Here's how the part is built. I have some questions about the finished solid (model axes, mm). A direction names the side the tool comes from. Coordinates: 2 decimals unless noted, no trailing zeros. Write each loop counter-clockwise with the first axis right and the second up, starting at its lowest first coordinate (ties: lowest second). Pieces come first, ordered by that corner, then holes.
Autodesk Fusion 360 part; units mm, degrees
sketch "Sketch1" plane through (0, 0, 0) normal (0, 0, 1) x (1, 0, 0)
  line L0 (0, 0) -> (47.5, 0)
  line L1 (47.5, 0) -> (47.5, 38)
  circle A0 centre (5, 33) radius 2.175
  line L2 (5, 33) -> (5, 26) construction
  circle A1 centre (5, 26) radius 2.25
  circle A2 centre (12.5, 26) radius 2.25
  circle A3 centre (12.5, 33) radius 2.175
  circle A4 centre (20, 26) radius 2.25
  circle A5 centre (20, 33) radius 2.175
  line L3 (5, 26) -> (5, 19) construction
  line L4 (5, 19) -> (5, 12) construction
  circle A6 centre (5, 19) radius 2.325
  circle A7 centre (5, 12) radius 2.4
  circle A8 centre (12.5, 19) radius 2.325
  circle A9 centre (12.5, 12) radius 2.4
  circle A10 centre (20, 19) radius 2.325
  circle A11 centre (20, 12) radius 2.4
  circle A12 centre (27.5, 26) radius 2.25
  circle A13 centre (27.5, 33) radius 2.175
  circle A14 centre (27.5, 19) radius 2.325
  circle A15 centre (27.5, 12) radius 2.4
  circle A16 centre (35, 26) radius 2.25
  circle A17 centre (35, 33) radius 2.175
  circle A18 centre (35, 19) radius 2.325
  circle A19 centre (35, 12) radius 2.4
  line L5 (5, 12) -> (5, 5) construction
  circle A20 centre (5, 5) radius 2.475
  circle A21 centre (12.5, 5) radius 2.475
  circle A22 centre (20, 5) radius 2.475
  circle A23 centre (27.5, 5) radius 2.475
  circle A24 centre (35, 5) radius 2.475
  circle A25 centre (42.5, 26) radius 2.25
  circle A26 centre (42.5, 33) radius 2.175
  circle A27 centre (42.5, 19) radius 2.325
  circle A28 centre (42.5, 12) radius 2.4
  circle A29 centre (42.5, 5) radius 2.475
  line L6 (47.5, 38) -> (0, 38)
  line L7 (0, 38) -> (0, 0)
  dimension "d2" = 4.35
  dimension "d4" = 4.5
  dimension "d7" = 7.5
  dimension "d8" = 0
  dimension "d13" = 4.65
  dimension "d14" = 4.8
  dimension "d21" = 4.95
  dimension "d27" = 5
  dimension "d28" = 5
  dimension "d29" = 5
  dimension "d30" = 5
sketch "Sketch2" plane through (0, 0, 0) normal (0, 0, 1) x (1, 0, 0)
  line L0 (47.5, 0) -> (47.5, 38)
  line L1 (0, 0) -> (47.5, 0)
  line L2 (47.5, 38) -> (0, 38)
  line L3 (0, 38) -> (0, 0)
extrude "Extrude1" add sketch "Sketch2" against normal blind 8
extrude "Extrude2" cut sketch "Sketch1" against normal blind 5.8 contours A0 | A1 | A6
extrude "Extrude3" cut sketch "Sketch1" against normal blind 5.8 draft -2 contours A2 | A3 | A8 | A9
extrude "Extrude4" cut sketch "Sketch1" against normal blind 5.7 draft -4 contours A4 | A5 | A10 | A11 | A22
extrude "Extrude5" cut sketch "Sketch1" against normal blind 5.8 draft -6 contours A12 | A14 | A15 | A23
extrude "Extrude6" cut sketch "Sketch1" against normal blind 5.8 draft -8 contours A18 | A19 | A24
extrude "Extrude7" cut sketch "Sketch1" against normal blind 5.8 draft -10 contours A28 | A29
fillet "Fillet1" radius 3 3 edges at (0, 0, -4) (47.5, 0, -4) (47.5, 38, -4)
equation "extrude_depth = 5.8 mm"
1) Will these pins go through, and if not, where does the flat tip stop? pin 1 (1.3 mm diameter, centred on x = 5.5, y = 26, fed in from +Z); pin 2 (6 mm diameter, centred on x = 12.5, y = 26.5, fed in from +Z); pin 3 (2 mm diameter, centred on x = 20, y = 5.5, fed in from +Z).
Values follow:
pin 1: stops at z = -5.8
pin 2: stops at z = 0
pin 3: stops at z = -5.7
2) I need wall thicknesses on probe 1 along Y at (x, z) = (5, -4) (3 decimals); probe 2 along Y at (x, z) = (44, -4.25); probe 3 along Z at (x, y) = (21, 18). Which ranges of each line are inside material? Lowest first, please.
Values follow:
probe 1: y = 0 to 16.675, 21.325 to 23.75, 28.25 to 30.825, 35.175 to 38
probe 2: y = 0 to 4.15, 5.85 to 11.31, 12.69 to 38
probe 3: z = -8 to -5.7
3) We'd pull the mould along X, two halves only. Please class faces 3 (the face through (5, 26, -5.8)), 4 (the face through (46.6, 37.14, -4.06)), 5 (the face through (27.061, 17.024, -2.859)): pulls with the +X half, pulls with the -X half, needs draft (parallel to the pull), parting line crosses it, or undercut.
Values follow:
face 3: undercut
face 4: pulls with the +X half
face 5: undercut
4) Imagine slicing it at C-C on z = -2. Count the separate pieces of the cut face and the enclosed holes in it, then the cut area to 3 significant figures.
Values follow:
separate pieces: 1
enclosed holes: 21
area: 1,490 mm2
5) Imagine slicing it at A-A on y = 5. Please give me the cut outline in (x, z) (3 decimals), then the cut area to 3 significant figures.
Values follow:
outline: (0, -8) - (47.5, -8) - (47.5, 0) - (44.975, 0) - (43.952, -5.8) - (41.048, -5.8) - (40.025, 0) - (37.475, 0) - (36.66, -5.8) - (33.34, -5.8) - (32.525, 0) - (29.975, 0) - (29.365, -5.8) - (25.635, -5.8) - (25.025, 0) - (22.475, 0) - (22.076, -5.7) - (17.924, -5.7) - (17.525, 0) - (0, 0) - close
area: 282 mm2
6) Imagine slicing it at D-D on y = 33. Please give me the cut outline in (x, z) (3 decimals).
Values follow:
outline: (0, -8) - (47.5, -8) - (47.5, 0) - (22.175, 0) - (21.776, -5.7) - (18.224, -5.7) - (17.825, 0) - (14.675, 0) - (14.472, -5.8) - (10.528, -5.8) - (10.325, 0) - (7.175, 0) - (7.175, -5.8) - (2.825, -5.8) - (2.825, 0) - (0, 0) - close
7) On a 3-axis mill with a long thin cutter (end or side, diameter ignored), from which of +Z, -Z, +X, -X, +Y, -Y can I reach the whole of each face in a straight line? I mean faces 1 (the face through (47.5, 19, -4)), 2 (the face through (10.85, 31.74, -2.86)). Say none if no direction works.
Values follow:
face 1: +Z, -Z, +X, +Y, -Y
face 2: +Z
8) Imagine slicing it at B-B on x = 27.5. Please give me the cut outline in (y, z) (3 decimals).
Values follow:
outline: (0, -8) - (38, -8) - (38, 0) - (28.25, 0) - (27.64, -5.8) - (24.36, -5.8) - (23.75, 0) - (21.325, 0) - (20.715, -5.8) - (17.285, -5.8) - (16.675, 0) - (14.4, 0) - (13.79, -5.8) - (10.21, -5.8) - (9.6, 0) - (7.475, 0) - (6.865, -5.8) - (3.135, -5.8) - (2.525, 0) - (0, 0) - close
